Geometry check sheet. Reference: the model listing, model coordinates, mm. Coordinates: 2 decimals unless noted, no trailing zeros. Write each loop counter-clockwise with the first axis right and the second up, starting at its lowest first coordinate (ties: lowest second). Pieces come first, ordered by that corner, then holes.
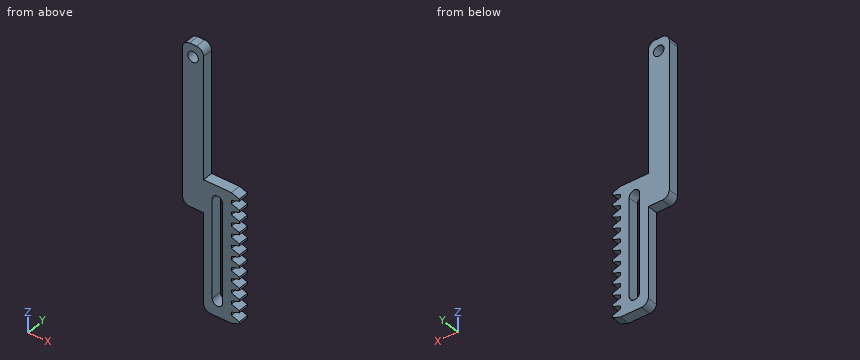
from build123d import *

# Parameters (mm, degrees)
CROQUIS1_R              = 1.5
SALIENTE_EXTRUIR2_DEPTH = 3


with BuildPart() as part:
    # Croquis1 → Saliente-Extruir2 (new body)
    with BuildSketch(Plane(origin=(0, 0, 0), x_dir=(1, 0, 0), z_dir=(0, 1, 0))):
        with BuildLine():
            Line((0.222991841, 27.097579335), (6.222991841, 27.097579335))
            Line((6.222991841, 27.097579335), (8.472991841, 26.278646308))
            Line((8.472991841, 26.278646308), (8.472991841, 25.663790451))
            Line((8.472991841, 25.663790451), (6.222991841, 24.844857424))
            Line((6.222991841, 24.844857424), (6.222991841, 23.955986685))
            Line((6.222991841, 23.955986685), (8.472991841, 23.137053658))
            Line((8.472991841, 23.137053658), (8.472991841, 22.522197801))
            Line((8.472991841, 22.522197801), (6.222991841, 21.703264774))
            Line((6.222991841, 21.703264774), (6.222991841, 20.814394035))
            Line((6.222991841, 20.814394035), (8.472991841, 19.995461008))
            Line((8.472991841, 19.995461008), (8.472991841, 19.380605151))
            Line((8.472991841, 19.380605151), (6.222991841, 18.561672124))
            Line((6.222991841, 18.561672124), (6.222991841, 17.672801385))
            Line((6.222991841, 17.672801385), (8.472991841, 16.853868358))
            Line((8.472991841, 16.853868358), (8.472991841, 16.239012501))
            Line((8.472991841, 16.239012501), (6.222991841, 15.420079474))
            Line((6.222991841, 15.420079474), (6.222991841, 14.531208735))
            Line((6.222991841, 14.531208735), (8.472991841, 13.712275708))
            Line((8.472991841, 13.712275708), (8.472991841, 13.097419851))
            Line((8.472991841, 13.097419851), (6.222991841, 12.278486824))
            Line((6.222991841, 12.278486824), (6.222991841, 11.389616085))
            Line((6.222991841, 11.389616085), (8.472991841, 10.570683058))
            Line((8.472991841, 10.570683058), (8.472991841, 9.955827201))
            Line((8.472991841, 9.955827201), (6.222991841, 9.136894174))
            Line((6.222991841, 9.136894174), (6.222991841, 8.248023435))
            Line((6.222991841, 8.248023435), (8.472991841, 7.429090408))
            Line((8.472991841, 7.429090408), (8.472991841, 6.814234551))
            Line((8.472991841, 6.814234551), (6.222991841, 5.995301524))
            Line((6.222991841, 5.995301524), (6.222991841, 5.106430785))
            Line((6.222991841, 5.106430785), (8.472991841, 4.287497758))
            Line((8.472991841, 4.287497758), (8.472991841, 3.672641901))
            Line((8.472991841, 3.672641901), (6.222991841, 2.853708874))
            Line((6.222991841, 2.853708874), (6.222991841, 1.964838135))
            Line((6.222991841, 1.964838135), (8.472991841, 1.145905108))
            Line((8.472991841, 1.145905108), (8.472991841, 0.531049251))
            Line((8.472991841, 0.531049251), (6.222991841, -0.287883776))
            Line((6.222991841, -0.287883776), (6.222991841, -1.176754515))
            Line((6.222991841, -1.176754515), (8.472991841, -1.995687542))
            Line((8.472991841, -1.995687542), (8.472991841, -2.610543399))
            Line((8.472991841, -2.610543399), (6.222991841, -3.429476426))
            Line((6.222991841, -3.429476426), (6.222991841, -4.318347165))
            Line((6.222991841, -4.318347165), (8.472991841, -5.137280192))
            Line((8.472991841, -5.137280192), (8.472991841, -5.752136049))
            Line((8.472991841, -5.752136049), (6.222991841, -6.571069076))
            Line((6.222991841, -6.571069076), (6.222991841, -7.459939815))
            Line((6.222991841, -7.459939815), (8.472991841, -8.278872842))
            Line((8.472991841, -8.278872842), (8.472991841, -8.893728699))
            Line((8.472991841, -8.893728699), (6.222991841, -9.712661726))
            Line((6.222991841, -9.712661726), (0.256792505, -9.712661726))
            Line((0.256792505, -9.712661726), (-1.743207495, -9.712661726))
            Line((-1.743207495, -9.712661726), (-1.743207495, -44.412661726))
            ThreePointArc((-1.743207495, -44.412661726), (-2.328993932, -45.826875288), (-3.743207495, -46.412661726))
            Line((-3.743207495, -46.412661726), (-5.743207495, -46.412661726))
            ThreePointArc((-5.743207495, -46.412661726), (-7.157421057, -45.826875288), (-7.743207495, -44.412661726))
            Line((-7.743207495, -44.412661726), (-7.743207495, -6.412661726))
            Line((-7.743207495, -6.412661726), (-7.743207495, -4.412661726))
            Line((-7.743207495, -4.412661726), (-7.743207495, -2.412661726))
            ThreePointArc((-7.743207495, -2.412661726), (-7.157421057, -0.998448163), (-5.743207495, -0.412661726))
            Line((-5.743207495, -0.412661726), (-1.743207495, -0.412661726))
            Line((-1.743207495, -0.412661726), (-1.743207495, 25.463721618))
            ThreePointArc((-1.743207495, 25.463721618), (-1.055232598, 26.635806328), (0.222991841, 27.097579335))
        make_face()
        with Locations((-4.743207495, -42.912661726)):
            Circle(CROQUIS1_R, mode=Mode.SUBTRACT)
        with BuildLine():
            Line((3.722991841, 22.597579335), (3.722991841, -5.402420665))
            ThreePointArc((3.722991841, -5.402420665), (2.222991841, -6.902420665), (0.722991841, -5.402420665))
            Line((0.722991841, -5.402420665), (0.722991841, 22.597579335))
            ThreePointArc((0.722991841, 22.597579335), (2.222991841, 24.097579335), (3.722991841, 22.597579335))
        make_face(mode=Mode.SUBTRACT)
    extrude(amount=SALIENTE_EXTRUIR2_DEPTH)


solid = part.part
1. Thickness scan on line 1 along X through (y, z) = (0.25, 31); line 2 along Z through (x, y) = (6, 2.5); line 3 along Z through (x, y) = (-5.75, 0.25). Record the ranges inside material, lowest first.
Computed values:
line 1: x = -7.74 to -1.74
line 2: z = -27.1 to 9.71
line 3: z = 0.41 to 41.8, 44.02 to 46.41
2. Sectioned sample at B-B, the plane x = 7.25. Give the number of separate pieces and of enclosed holes in the cut face, and give its area (3 significant figures).
Computed values:
separate pieces: 12
enclosed holes: 0
area: 54.2 mm2
3. Gauge pin test, flat ends, axial feed: pin 1 Ø0.9 at (x, y) = (-4.5, 1.5) entering from -Z; pin 2 Ø6 at (x, z) = (1, 37.5) entering from +Y; pin 3 Ø1.5 at (x, y) = (1, 2.5) entering from +Z. Record the tip position at first contact, or that the pin passes through.
Computed values:
pin 1: stops at z = 0.41
pin 2: stops at y = 3
pin 3: stops at z = 9.71
4. Sectioned sample at A-A, the plane x = 1.5. Record the boundary of the cut face in (y, z).
Computed values:
outline: (0, -27.1) - (3, -27.1) - (3, -23.91) - (0, -23.91) - close; (0, 6.72) - (3, 6.72) - (3, 9.71) - (0, 9.71) - close
5. Sectioned sample at D-D, the plane z = 21.5. Record the boundary of the cut face in (x, y), and give its area (3 significant figures).
Computed values:
outline: (-7.74, 0) - (-1.74, 0) - (-1.74, 3) - (-7.74, 3) - close
area: 18.0 mm2
